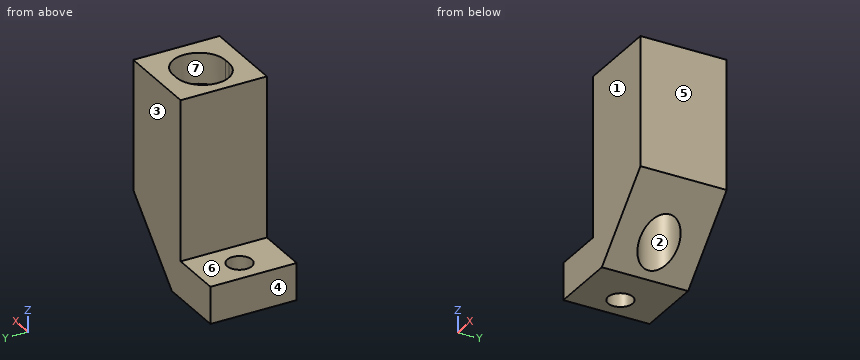
```python
from build123d import *

# Parameters (mm, degrees)
PAD002_DEPTH     = 7
POCKET003_DEPTH  = 5
HOLE_D           = 3.4
HOLE_CBORE_D     = 6.1
HOLE_CBORE_DEPTH = 20
SKETCH007_R      = 2
POCKET004_DEPTH  = 6


with BuildPart() as part:
    # Sketch005 → Pad002 (new body, symmetric)
    with BuildSketch(Plane.XZ.offset(2)):
        Polygon((43, -13), (43, -19), (54, -19), (65, -8), (65, 13), (51.500001, 13), (51.500001, -13), align=None)
    extrude(amount=PAD002_DEPTH, both=True)

    # Sketch008 → Pocket003 (cut)
    with BuildSketch(Plane(origin=(0, 0, 13), x_dir=(-1, 0, 0), z_dir=(0, 0, 1))):
        with BuildLine():
            ThreePointArc((-57.501297, -2.25), (-53.251297, 2), (-57.501297, 6.25))
            Line((-57.501297, 6.25), (-58.500001, 6.25))
            ThreePointArc((-58.500001, 6.25), (-62.750001, 2), (-58.500001, -2.25))
            Line((-58.500001, -2.25), (-57.501297, -2.25))
        make_face()
    extrude(amount=-POCKET003_DEPTH, mode=Mode.SUBTRACT)

    # Hole (through all)
    with Locations(Plane(origin=(0, 0, -19), x_dir=(1, 0, 0), z_dir=(0, 0, -1))):
        with Locations((58, 2)):
            CounterBoreHole(HOLE_D / 2, HOLE_CBORE_D / 2, HOLE_CBORE_DEPTH)

    # Sketch007 (on Face2 of Pad002) → Pocket004 (cut)
    with BuildSketch(Plane(origin=(0, 0, -19), x_dir=(1, 0, 0), z_dir=(0, 0, -1))):
        with Locations((47, 2)):
            Circle(SKETCH007_R)
    extrude(amount=-POCKET004_DEPTH, mode=Mode.SUBTRACT)


with BuildPart() as part_1:
    # Body001 placement: moved
    add(part.part.moved(Location((0, -40, 0))))


solid = part_1.part
```
CAD build for the part. Positions are in the model's coordinates, mm. Face numbers are marked on the shaded views. A direction names the side the tool comes from. Coordinates: 2 decimals unless noted, no trailing zeros. Order: outer loops, then holes, each group sorted by start corner. A loop starts at its lowest first (then second) coordinate and runs counter-clockwise, first axis right, second up. Notation, with made-up numbers: M 10.25,-4 L 35.25,-4 A25 cw 35.25,16 Z; hole C 25,60 d6. An arc over 180 degrees is marked long. Write each question's results on one line, items separated by ' | '. Start each with the question number.
Q1. Cut at C-C (z = 5). List the corners of the cut face in (x, y).
Q2. Pull direction Y, two halves, no side cores. Call the marked faces 1, 2, 3 and 4: +Y half, -Y half, draft (parallel to the pull), parting line (faces both ways), or undercut.
Q3. Cut at B-B (x = 47). List the corners of the cut face in (y, z).
Q4. Cut at D-D (y = -36). List the corners of the cut face in (x, z).
Q5. Flat gauge pins, fed straight in: P1, Ø5, axis at x = 47, y = -42, coming from the -Z side; P2, Ø7, axis at y = -43.5, z = 6, coming from the -X side; P3, Ø5, axis at x = 59, y = -43, coming from the -Z side; P4, Ø4, axis at x = 56, y = -43.5, coming from the +Z side. Where does each tip first touch, or does it go through?
Q6. Drill centre lines: probe 1 along X at (y, z) = (-42, 5.5); probe 2 along X at (y, z) = (-42, -15.5); probe 3 along Y at (x, z) = (58, 6.25). Where is each one in solid material? Low to high. Write a range as from..to.
Q7. Cut at A-A (y = -42). List the corners of the cut face in (x, z).
Q8. Which spindle directions (+Z, -Z, +X, -X, +Y, -Y) get a long thin tool onto all of the face, cutting with end or side? Do the marked faces 5, 6 and 7. Say none if no direction does.
Found:
1) outline: M 51.5,-49 L 65,-49 L 65,-35 L 51.5,-35 Z; hole C 58,-42 d3.4
2) face 1: -Y half | face 2: undercut | face 3: +Y half | face 4: draft
3) outline: M -49,-19 L -44,-19 L -44,-13 L -49,-13 Z; M -40,-19 L -35,-19 L -35,-13 L -40,-13 Z
4) outline: M 43,-19 L 54,-19 L 65,-8 L 65,13 L 51.5,13 L 51.5,-13 L 43,-13 Z
5) P1: z = -19 | P2: x = 51.5 | P3: z = -15.48 | P4: z = 8
6) probe 1: 51.5..56.3, 59.7..65 | probe 2: 43..45, 49..54.95 | probe 3: -49..-43.7, -40.3..-35
7) outline: M 43,-19 L 45,-19 L 45,-13 L 43,-13 Z; M 49,-19 L 54,-19 L 54.95,-18.05 L 54.95,1 L 56.3,1 L 56.3,8 L 53.25,8 L 53.25,13 L 51.5,13 L 51.5,-13 L 49,-13 Z; M 59.7,1 L 61.05,1 L 61.05,-11.95 L 65,-8 L 65,13 L 62.75,13 L 62.75,8 L 59.7,8 Z
8) face 5: +Z, -Z, +X, +Y, -Y | face 6: +Z, -X, +Y, -Y | face 7: +Z
